Work out the finished part from the listing and answer in its coordinate system (mm). Face numbers are marked on the shaded views. A direction names the side the tool comes from. Coordinates: 2 decimals unless noted, no trailing zeros. Order: outer loops, then holes, each group sorted by start corner. A loop starts at its lowest first (then second) coordinate and runs counter-clockwise, first axis right, second up. Notation, with made-up numbers: M 22.25,-27.75 L 64.25,-27.75 A38 cw 64.25,10.25 Z; hole C 79.25,-37 d5. An arc over 180 degrees is marked long. Use a Markdown table: item, result.
from build123d import *

# Parameters (mm, degrees)
SKETCH_1_W          = 165
SKETCH_1_H          = 45
SKETCH_1_R          = 1.75
SKETCH_1_R_2        = 2.55
SKETCH_1_W_2        = 105.5
SKETCH_1_H_2        = 2.5
EXTRUDE_2_DEPTH     = 3
SKETCH_1_5_R        = 2.75
SKETCH_1_5_R_2      = 1.75
CUT_EXTRUDE_2_DEPTH = 1.2
SKETCH_1_7_W        = 105.5
SKETCH_1_7_H        = 2.5
EXTRUDE_3_DEPTH     = 38
FILLET_1_R          = 5
FILLET_2_R          = 1
SKETCH_3D_1_R       = 1.6
CUT_EXTRUDE_3_DEPTH = 2.5
EXTRUDE_5_DEPTH     = 3


with BuildPart() as part:
    # 草图1 → 凸台-拉伸2 (new body)
    with BuildSketch(Plane.XY):
        with Locations((12.080789946, 2.099629791)):
            Rectangle(SKETCH_1_W, SKETCH_1_H)
        with Locations((-65.919210054, 20.099629791)):
            Circle(SKETCH_1_R, mode=Mode.SUBTRACT)
        with Locations((-65.919210054, -15.900370209)):
            Circle(SKETCH_1_R, mode=Mode.SUBTRACT)
        with Locations((90.080789946, -15.900370209)):
            Circle(SKETCH_1_R, mode=Mode.SUBTRACT)
        with Locations((90.080789946, 20.099629791)):
            Circle(SKETCH_1_R, mode=Mode.SUBTRACT)
        with Locations((12.17205321, 3.14535325)):
            Circle(SKETCH_1_R_2, mode=Mode.SUBTRACT)
        with BuildLine():
            Line((25.580789946, 12.599629791), (63.580789946, 12.599629791))
            ThreePointArc((63.580789946, 12.599629791), (64.287896727, 12.306736572), (64.580789946, 11.599629791))
            Line((64.580789946, 11.599629791), (64.580789946, 10.599629791))
            ThreePointArc((64.580789946, 10.599629791), (64.287896727, 9.89252301), (63.580789946, 9.599629791))
            Line((63.580789946, 9.599629791), (25.580789946, 9.599629791))
            ThreePointArc((25.580789946, 9.599629791), (24.873683165, 9.89252301), (24.580789946, 10.599629791))
            Line((24.580789946, 10.599629791), (24.580789946, 11.599629791))
            ThreePointArc((24.580789946, 11.599629791), (24.873683165, 12.306736572), (25.580789946, 12.599629791))
        make_face(mode=Mode.SUBTRACT)
        with BuildLine():
            Line((-39.419210054, 12.599629791), (-1.419210054, 12.599629791))
            ThreePointArc((-1.419210054, 12.599629791), (-0.712103273, 12.306736572), (-0.419210054, 11.599629791))
            Line((-0.419210054, 11.599629791), (-0.419210054, 10.599629791))
            ThreePointArc((-0.419210054, 10.599629791), (-0.712103273, 9.89252301), (-1.419210054, 9.599629791))
            Line((-1.419210054, 9.599629791), (-39.419210054, 9.599629791))
            ThreePointArc((-39.419210054, 9.599629791), (-40.126316835, 9.89252301), (-40.419210054, 10.599629791))
            Line((-40.419210054, 10.599629791), (-40.419210054, 11.599629791))
            ThreePointArc((-40.419210054, 11.599629791), (-40.126316835, 12.306736572), (-39.419210054, 12.599629791))
        make_face(mode=Mode.SUBTRACT)
        with BuildLine():
            Line((25.580789946, 6.599629791), (63.580789946, 6.599629791))
            ThreePointArc((63.580789946, 6.599629791), (64.287896727, 6.306736572), (64.580789946, 5.599629791))
            Line((64.580789946, 5.599629791), (64.580789946, 4.599629791))
            ThreePointArc((64.580789946, 4.599629791), (64.287896727, 3.89252301), (63.580789946, 3.599629791))
            Line((63.580789946, 3.599629791), (25.580789946, 3.599629791))
            ThreePointArc((25.580789946, 3.599629791), (24.873683165, 3.89252301), (24.580789946, 4.599629791))
            Line((24.580789946, 4.599629791), (24.580789946, 5.599629791))
            ThreePointArc((24.580789946, 5.599629791), (24.873683165, 6.306736572), (25.580789946, 6.599629791))
        make_face(mode=Mode.SUBTRACT)
        with BuildLine():
            Line((25.580789946, 0.599629791), (63.580789946, 0.599629791))
            ThreePointArc((63.580789946, 0.599629791), (64.287896727, 0.306736572), (64.580789946, -0.400370209))
            Line((64.580789946, -0.400370209), (64.580789946, -1.400370209))
            ThreePointArc((64.580789946, -1.400370209), (64.287896727, -2.10747699), (63.580789946, -2.400370209))
            Line((63.580789946, -2.400370209), (25.580789946, -2.400370209))
            ThreePointArc((25.580789946, -2.400370209), (24.873683165, -2.10747699), (24.580789946, -1.400370209))
            Line((24.580789946, -1.400370209), (24.580789946, -0.400370209))
            ThreePointArc((24.580789946, -0.400370209), (24.873683165, 0.306736572), (25.580789946, 0.599629791))
        make_face(mode=Mode.SUBTRACT)
        with BuildLine():
            Line((25.580789946, -5.400370209), (63.580789946, -5.400370209))
            ThreePointArc((63.580789946, -5.400370209), (64.287896727, -5.693263428), (64.580789946, -6.400370209))
            Line((64.580789946, -6.400370209), (64.580789946, -7.400370209))
            ThreePointArc((64.580789946, -7.400370209), (64.287896727, -8.10747699), (63.580789946, -8.400370209))
            Line((63.580789946, -8.400370209), (25.580789946, -8.400370209))
            ThreePointArc((25.580789946, -8.400370209), (24.873683165, -8.10747699), (24.580789946, -7.400370209))
            Line((24.580789946, -7.400370209), (24.580789946, -6.400370209))
            ThreePointArc((24.580789946, -6.400370209), (24.873683165, -5.693263428), (25.580789946, -5.400370209))
        make_face(mode=Mode.SUBTRACT)
        with BuildLine():
            Line((-39.419210054, 6.599629791), (-1.419210054, 6.599629791))
            ThreePointArc((-1.419210054, 6.599629791), (-0.712103273, 6.306736572), (-0.419210054, 5.599629791))
            Line((-0.419210054, 5.599629791), (-0.419210054, 4.599629791))
            ThreePointArc((-0.419210054, 4.599629791), (-0.712103273, 3.89252301), (-1.419210054, 3.599629791))
            Line((-1.419210054, 3.599629791), (-39.419210054, 3.599629791))
            ThreePointArc((-39.419210054, 3.599629791), (-40.126316835, 3.89252301), (-40.419210054, 4.599629791))
            Line((-40.419210054, 4.599629791), (-40.419210054, 5.599629791))
            ThreePointArc((-40.419210054, 5.599629791), (-40.126316835, 6.306736572), (-39.419210054, 6.599629791))
        make_face(mode=Mode.SUBTRACT)
        with BuildLine():
            Line((-39.419210054, 0.599629791), (-1.419210054, 0.599629791))
            ThreePointArc((-1.419210054, 0.599629791), (-0.712103273, 0.306736572), (-0.419210054, -0.400370209))
            Line((-0.419210054, -0.400370209), (-0.419210054, -1.400370209))
            ThreePointArc((-0.419210054, -1.400370209), (-0.712103273, -2.10747699), (-1.419210054, -2.400370209))
            Line((-1.419210054, -2.400370209), (-39.419210054, -2.400370209))
            ThreePointArc((-39.419210054, -2.400370209), (-40.126316835, -2.10747699), (-40.419210054, -1.400370209))
            Line((-40.419210054, -1.400370209), (-40.419210054, -0.400370209))
            ThreePointArc((-40.419210054, -0.400370209), (-40.126316835, 0.306736572), (-39.419210054, 0.599629791))
        make_face(mode=Mode.SUBTRACT)
        with BuildLine():
            Line((-39.419210054, -5.400370209), (-1.419210054, -5.400370209))
            ThreePointArc((-1.419210054, -5.400370209), (-0.712103273, -5.693263428), (-0.419210054, -6.400370209))
            Line((-0.419210054, -6.400370209), (-0.419210054, -7.400370209))
            ThreePointArc((-0.419210054, -7.400370209), (-0.712103273, -8.10747699), (-1.419210054, -8.400370209))
            Line((-1.419210054, -8.400370209), (-39.419210054, -8.400370209))
            ThreePointArc((-39.419210054, -8.400370209), (-40.126316835, -8.10747699), (-40.419210054, -7.400370209))
            Line((-40.419210054, -7.400370209), (-40.419210054, -6.400370209))
            ThreePointArc((-40.419210054, -6.400370209), (-40.126316835, -5.693263428), (-39.419210054, -5.400370209))
        make_face(mode=Mode.SUBTRACT)
        with BuildLine():
            Line((7.580789946, -10.400370209), (16.580789946, -10.400370209))
            ThreePointArc((16.580789946, -10.400370209), (16.934343337, -10.546816818), (17.080789946, -10.900370209))
            Line((17.080789946, -10.900370209), (17.080789946, -13.900370209))
            ThreePointArc((17.080789946, -13.900370209), (16.934343337, -14.253923599), (16.580789946, -14.400370209))
            Line((16.580789946, -14.400370209), (7.580789946, -14.400370209))
            ThreePointArc((7.580789946, -14.400370209), (7.227236556, -14.253923599), (7.080789946, -13.900370209))
            Line((7.080789946, -13.900370209), (7.080789946, -10.900370209))
            ThreePointArc((7.080789946, -10.900370209), (7.227236556, -10.546816818), (7.580789946, -10.400370209))
        make_face(mode=Mode.SUBTRACT)
        with Locations((12.330789946, -18.650370209)):
            Rectangle(SKETCH_1_W_2, SKETCH_1_H_2, mode=Mode.SUBTRACT)
    extrude(amount=EXTRUDE_2_DEPTH)

    # 草图1<5> → 切除-拉伸2 (cut)
    # profile 1 of 4: a face of its own
    with BuildSketch(Plane.XY):
        with Locations((90.080789946, 20.099629791)):
            Circle(SKETCH_1_5_R)
        with Locations((90.080789946, 20.099629791)):
            Circle(SKETCH_1_5_R_2, mode=Mode.SUBTRACT)
    # profile 2 of 4: a face of its own
    with BuildSketch(Plane.XY):
        with Locations((90.080789946, -15.900370209)):
            Circle(SKETCH_1_5_R)
        with Locations((90.080789946, -15.900370209)):
            Circle(SKETCH_1_5_R_2, mode=Mode.SUBTRACT)
    # profile 3 of 4: a face of its own
    with BuildSketch(Plane.XY):
        with Locations((-65.919210054, 20.099629791)):
            Circle(SKETCH_1_5_R)
        with Locations((-65.919210054, 20.099629791)):
            Circle(SKETCH_1_5_R_2, mode=Mode.SUBTRACT)
    # profile 4 of 4: a face of its own
    with BuildSketch(Plane.XY):
        with Locations((-65.919210054, -15.900370209)):
            Circle(SKETCH_1_5_R)
        with Locations((-65.919210054, -15.900370209)):
            Circle(SKETCH_1_5_R_2, mode=Mode.SUBTRACT)
    extrude(amount=CUT_EXTRUDE_2_DEPTH, mode=Mode.SUBTRACT)

    # 草图1<7> → 凸台-拉伸3 (add)
    with BuildSketch(Plane.XY):
        with Locations((12.330789946, -18.650370209)):
            Rectangle(SKETCH_1_7_W, SKETCH_1_7_H)
    extrude(amount=EXTRUDE_3_DEPTH)

    # 圆角1
    fillet_1_edges = [part.edges().sort_by_distance(p)[0] for p in [
        (65.080789946, -18.650370209, 38),
        (-40.419210054, -18.650370209, 38),
    ]]
    fillet(fillet_1_edges, radius=FILLET_1_R)

    # 圆角2
    fillet_2_edges = [part.edges().sort_by_distance(p)[0] for p in [
        (94.580789946, -20.400370209, 1.5),
        (-70.419210054, -20.400370209, 1.5),
        (-70.419210054, 24.599629791, 1.5),
        (94.580789946, 24.599629791, 1.5),
    ]]
    fillet(fillet_2_edges, radius=FILLET_2_R)

    # Sketch 3D_1 → 切除-拉伸3 (cut)
    with BuildSketch(Plane(origin=(-27.669210054, -17.400370209, 5.5), x_dir=(0.9363291775690445, 0, 0.35112344158839165), z_dir=(0, -1, 0))):
        with Locations(Location((0, 0, 0), (0, 0, 159.44395478))):
            Circle(SKETCH_3D_1_R)
        with Locations(Location((74.906334206, -28.089875327, 0), (0, 0, 159.44395478))):
            Circle(SKETCH_3D_1_R)
        with Locations(Location((10.533703248, 28.089875327, 0), (0, 0, 159.44395478))):
            Circle(SKETCH_3D_1_R)
        with Locations(Location((85.440037453, 0, 0), (0, 0, 159.44395478))):
            Circle(SKETCH_3D_1_R)
    extrude(amount=CUT_EXTRUDE_3_DEPTH, mode=Mode.SUBTRACT)

    # 草图1<10> → 凸台-拉伸5 (add)
    with BuildSketch(Plane.XY):
        with BuildLine():
            Line((10.14705321, 4.695151624), (14.19705321, 4.695151624))
            ThreePointArc((14.19705321, 4.695151624), (12.17205321, 5.69535325), (10.14705321, 4.695151624))
        make_face()
        with BuildLine():
            ThreePointArc((10.14705321, 1.595554876), (12.17205321, 0.59535325), (14.19705321, 1.595554876))
            Line((14.19705321, 1.595554876), (10.14705321, 1.595554876))
        make_face()
    extrude(amount=EXTRUDE_5_DEPTH)


solid = part.part
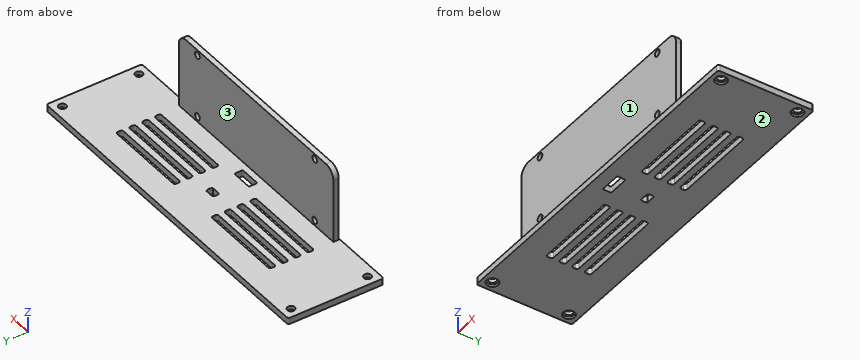
1. For the marked faces 1, 2 and 3, determine the directions among +Z, -Z, +X, -X, +Y, -Y from which every point of the face is accessible in a straight line to the end or side of a thin tool.
Answers below:
| item | result |
|---|---|
| face 1 | +Z, +X, -X, -Y |
| face 2 | -Z, +X, -X, +Y, -Y |
| face 3 | +Z, +X, -X, +Y |
2. Section D-D on z = 35.5 is taken. Determine the outline of the cut face in (x, y), then the cut area to 3 significant figures.
Answers below:
| item | result |
|---|---|
| outline | M -39.75,-19.9 L -29.27,-19.9 L -29.27,-17.4 L -39.75,-17.4 Z; M -26.07,-19.9 L 50.73,-19.9 L 50.73,-17.4 L -26.07,-17.4 Z; M 53.93,-19.9 L 64.41,-19.9 L 64.41,-17.4 L 53.93,-17.4 Z |
| area | 244 mm² |
3. Section A-A on z = 5.5 is taken. Determine the outline of the cut face in (x, y).
Answers below:
| item | result |
|---|---|
| outline | M -40.42,-19.9 L -29.27,-19.9 L -29.27,-17.4 L -40.42,-17.4 Z; M -26.07,-19.9 L 50.73,-19.9 L 50.73,-17.4 L -26.07,-17.4 Z; M 53.93,-19.9 L 65.08,-19.9 L 65.08,-17.4 L 53.93,-17.4 Z |
4. Section B-B on x = 28 is taken. Determine the outline of the cut face in (y, z), then the cut area to 4 significant figures.
Answers below:
| item | result |
|---|---|
| outline | M -20.4,0 L -8.4,0 L -8.4,3 L -17.4,3 L -17.4,38 L -19.9,38 L -19.9,3 L -20.4,3 Z; M -5.4,0 L -2.4,0 L -2.4,3 L -5.4,3 Z; M 0.6,0 L 3.6,0 L 3.6,3 L 0.6,3 Z; M 6.6,0 L 9.6,0 L 9.6,3 L 6.6,3 Z; M 12.6,0 L 24.6,0 L 24.6,3 L 12.6,3 Z |
| area | 186.5 mm² |
5. Find the intervals of material crossed by probe 1 along Y at (x, z) = (0.5, 28); probe 2 along Z at (x, y) = (16.5, 1.5); probe 3 along X at (y, z) = (-18, 12.5), in increasing order.
Answers below:
| item | result |
|---|---|
| probe 1 | -19.9 to -17.4 |
| probe 2 | 0 to 3 |
| probe 3 | -40.42 to 65.08 |
6. Flat-ended cylindrical pins translate along their axes: P1, Ø8, axis at x = 34, y = 6, coming from the +Z side; P2, Ø3, axis at y = -18, z = 13.5, coming from the +X side; P3, Ø3, axis at x = -8, z = 14.5, coming from the -Y side. Find the tip coordinate at first contact, or state that the pin passes through.
Answers below:
| item | result |
|---|---|
| P1 | z = 3 |
| P2 | x = 65.08 |
| P3 | y = -19.9 |
7. Section C-C on z = 24 is taken. Determine the outline of the cut face in (x, y), then the cut area to 3 significant figures.
Answers below:
| item | result |
|---|---|
| outline | M -40.42,-19.9 L 65.08,-19.9 L 65.08,-17.4 L -40.42,-17.4 Z |
| area | 264 mm² |
